Geometry: final body of the model. Coordinates: model frame, mm. A direction names the side the tool comes from. Give positions to 0.01 mm unless a question says otherwise; leave off trailing zeros. Order: outer loops, then holes, each group sorted by start corner. A loop starts at its lowest first (then second) coordinate and runs counter-clockwise, first axis right, second up. Notation, with made-up numbers: (38.25, 30.5) - (85.25, 30.5) arc R7 ccw to (85.25, 39.5) - close; hole circle Ø4 at (-14, -28). An arc over 180 degrees is marked (long way). One line per question, with ' | ' between items. Start each with the question number.
from build123d import *

# Parameters (mm, degrees)
SKETCH1_W           = 20
SKETCH1_H           = 20
BOSS_EXTRUDE1_DEPTH = 1
BOSS_EXTRUDE2_DEPTH = 2.1
CHAMFER1_SIZE       = 0.5
SKETCH3_W           = 20
SKETCH3_H           = 20
BOSS_EXTRUDE3_DEPTH = 2.1


with BuildPart() as part:
    # Sketch1 → Boss-Extrude1 (new body)
    with BuildSketch(Plane(origin=(0, 0, 0), x_dir=(1, 0, 0), z_dir=(0, 1, 0))):
        with Locations((10, 10)):
            Rectangle(SKETCH1_W, SKETCH1_H)
    extrude(amount=BOSS_EXTRUDE1_DEPTH)

    # Sketch2 → Boss-Extrude2 (add)
    with BuildSketch(Plane(origin=(0, 1, 0), x_dir=(1, 0, 0), z_dir=(0, 1, 0))):
        Polygon((18, 15.5), (20, 15.5), (20, 20), (0, 20), (0, 0), (20, 0), (20, 4.5), (18, 4.5), (18, 1.95), (2, 1.95), (2, 18.05), (18, 18.05), align=None)
    extrude(amount=BOSS_EXTRUDE2_DEPTH)

    # Chamfer1
    chamfer1_edges = [part.edges().sort_by_distance(p)[0] for p in [
        (20, 1, -10),
    ]]
    chamfer(chamfer1_edges, length=CHAMFER1_SIZE)

    # Sketch3 → Boss-Extrude3 (add)
    with BuildSketch(Plane(origin=(0, 3.1, 0), x_dir=(1, 0, 0), z_dir=(0, 1, 0))):
        with Locations((10, 10)):
            Rectangle(SKETCH3_W, SKETCH3_H)
    extrude(amount=BOSS_EXTRUDE3_DEPTH)


solid = part.part
(1) Cut plane B-B, the plane y = 2.45. Return the cut outline in (x, z).
(2) Contact query for a flat-ended pin moving along its axis: P1, Ø1.7, axis at y = 2, z = -9.5, coming from the +X side. Output: stop coordinate, or through.
(3) Cut plane D-D, the plane z = -2.75. Return the cut outline in (x, y).
(4) Material intervals for line 1 along Y through (x, z) = (10.75, -3); line 2 along Z through (x, y) = (11.25, 2.45); line 3 along X through (y, z) = (1.2, -17.75), sorted ascending. Write a range as from..to.
(5) Pull-direction query (Z, two-part tool) for faces 1 (the flat face through (10, 3, 0)), 2 (the flat face through (20, 4, -10)), 3 (the flat face through (11, 1, -10)); classes: +Z half, -Z half, draft (parallel to the pull), parting line (faces both ways), or undercut.
(6) Cut plane A-A, the plane x = 12.25. Return the cut outline in (y, z).
(7) Cut plane C-C, the plane z = -12.5. Return the cut outline in (x, y).
(8) Access query for faces 4 (the flat face through (10, 0, -10)), 5 (the flat face through (2, 2, -10)), 6 (the flat face through (19, 2, -4.5)). Directions: +Z, -Z, +X, -X, +Y, -Y. A direction counts if a zero-diameter tool reaches every point of the face in a straight line with its end or side. Return the directions, or none.
Results are:
1) outline: (0, -20) - (20, -20) - (20, -15.5) - (18, -15.5) - (18, -18.05) - (2, -18.05) - (2, -1.95) - (18, -1.95) - (18, -4.5) - (20, -4.5) - (20, 0) - (0, 0) - close
2) P1: x = 2
3) outline: (0, 0) - (20, 0) - (20, 5.2) - (0, 5.2) - close; hole (2, 1) - (18, 1) - (18, 3.1) - (2, 3.1) - close
4) line 1: 0..1, 3.1..5.2 | line 2: -20..-18.05, -1.95..0 | line 3: 0..2, 18..20
5) face 1: +Z half | face 2: draft | face 3: undercut
6) outline: (0, -20) - (5.2, -20) - (5.2, 0) - (0, 0) - close; hole (1, -18.05) - (3.1, -18.05) - (3.1, -1.95) - (1, -1.95) - close
7) outline: (0, 0) - (20, 0) - (20, 0.5) - (19.5, 1) - (2, 1) - (2, 3.1) - (20, 3.1) - (20, 5.2) - (0, 5.2) - close
8) face 4: +Z, -Z, +X, -X, -Y | face 5: none | face 6: +X
